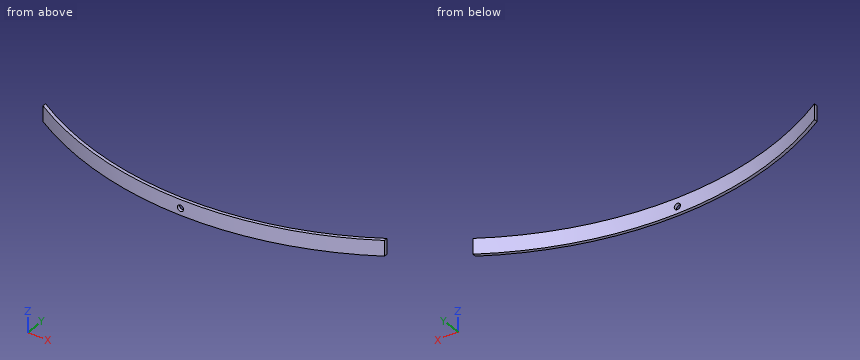
```python
from build123d import *

# Parameters (mm, degrees)
BOSS_EXTRUDE1_DEPTH = 50
SKETCH3_R           = 10
CUT_EXTRUDE1_DEPTH  = 1205.117934423


with BuildPart() as part:
    # Sketch1 → Boss-Extrude1 (new body)
    with BuildSketch(Plane.XY):
        with BuildLine():
            Line((-550, -906.145683651), (-550, -917.823512447))
            ThreePointArc((-550, -917.823512447), (0, -1070), (550, -917.823512447))
            Line((550, -917.823512447), (550, -906.145683651))
            ThreePointArc((550, -906.145683651), (0, -1060), (-550, -906.145683651))
        make_face()
    extrude(amount=BOSS_EXTRUDE1_DEPTH)

    # Sketch3 → Cut-Extrude1 (cut, through all)
    with BuildSketch(Plane(origin=(0, 0, 0), x_dir=(1, 0, 0), z_dir=(0, 1, 0))):
        with Locations(Location((0, -22.5, 0), (0, 0, 270))):
            Circle(SKETCH3_R)
    extrude(amount=-CUT_EXTRUDE1_DEPTH, mode=Mode.SUBTRACT)


solid = part.part
```
Can you work these out from the model? Positions are in its coordinate system, mm. Give positions to 0.01 mm unless a question says otherwise; leave off trailing zeros. Write each loop counter-clockwise with the first axis right and the second up, starting at its lowest first coordinate (ties: lowest second). Pieces come first, ordered by that corner, then holes. Notation, with made-up numbers: (37, 60.25) -> (68, 60.25) arc R8 cw to (68, 72.25) -> close; hole circle Ø11 at (-4, 38.5). An arc over 180 degrees is marked (long way). Write item = value, one per line.
(1) Suppose I cut it at D-D on x = 115. Write out the boundary of the cut face in (y, z).
Worked out:
outline = (-1063.8, 0) -> (-1053.74, 0) -> (-1053.74, 50) -> (-1063.8, 50) -> close
(2) Suppose I cut it at B-B on z = 22.5. Write out the boundary of the cut face in (x, y).
Worked out:
outline = (-550, -917.82) arc R1070 ccw to (-10, -1069.95) -> (-10, -1059.95) arc R1060 cw to (-550, -906.15) -> close; (10, -1069.95) arc R1070 ccw to (550, -917.82) -> (550, -906.15) arc R1060 cw to (10, -1059.95) -> close
(3) Suppose I cut it at A-A on x = 0. Write out the boundary of the cut face in (y, z), then the cut area to 3 significant figures.
Worked out:
outline = (-1070, 0) -> (-1060, 0) -> (-1060, 12.5) -> (-1070, 12.5) -> close; (-1070, 32.5) -> (-1060, 32.5) -> (-1060, 50) -> (-1070, 50) -> close
area = 300 mm^2
(4) Suppose I cut it at C-C on x = -303. Write out the boundary of the cut face in (y, z), then the cut area to 3 significant figures.
Worked out:
outline = (-1026.2, 0) -> (-1015.77, 0) -> (-1015.77, 50) -> (-1026.2, 50) -> close
area = 522 mm^2
(5) I need wall thicknesses on probe 1 along Z at (x, y) = (0, -1066); probe 2 along X at (y, z) = (-944, 47.5); probe 3 along Y at (x, z) = (-482, 3). Which ranges of each line are inside material? Lowest first, please. Write a range as from..to.
Worked out:
probe_1 = 0..12.5, 32.5..50
probe_2 = -503.75..-482.15, 482.15..503.75
probe_3 = -955.29..-944.07
(6) I'm going to push flat-ended pins straight in: P1, Ø12, axis at y = -971.5, z = 7.5, coming from the +X side; P2, Ø2, axis at y = -925.5, z = 22, coming from the -X side; P3, Ø3, axis at y = -931, z = 23, coming from the +X side; P4, Ø16, axis at x = 0, z = 22.5, coming from the -Y side (1 decimal). Where does each tip first touch, or does it pass through?
Worked out:
P1 = 461.2
P2 = -538.7
P3 = 530.03
P4 = through
